Work out the finished part from the listing and answer in its coordinate system (mm). A direction names the side the tool comes from. Coordinates: 2 decimals unless noted, no trailing zeros. Loops run counter-clockwise (first coordinate to the right, second up) from the corner with the lowest first, then second, coordinate; pieces in that order, holes last. Notation, with made-up numbers: (71, 56) -> (85, 56) arc R12 ccw to (85, 68) -> close; hole circle Ø5 at (6, 18.25). An arc over 180 degrees is marked (long way). One line per question, with ' | ' between items.
```python
from build123d import *

# Parameters (mm, degrees)
F0_R          = 12.7
F1_DEPTH      = 25.4
F2_R          = 12.7
F3_R          = 12.69999
F4_R          = 17.8783824342
F5_DEPTH      = 1.27
F5_DEPTH_BACK = 2.032
F6_R          = 10.795
F7_DEPTH      = 38.1
F8_R          = 19.05
F9_DEPTH      = 15.24


# Not quite as in the source:
# - a fillet or chamfer that OpenCascade refuses, or shapes differently, is made with other operations: its cross-section is extruded or revolved along the edge and cut away or added
# - a fillet or chamfer is up to 0.001 mm smaller than in the source, because OpenCascade refuses the exact size


with BuildPart() as f1:
    # F0 (on Front) → F1 (new body)
    with BuildSketch(Plane.XZ):
        Circle(F0_R)
    extrude(amount=F1_DEPTH)

    # F2
    f2_edges = [f1.edges().sort_by_distance(p)[0] for p in [
        (-12.7, -25.4, 0),
    ]]
    fillet(f2_edges, radius=F2_R)

    # F3 (radius 12.7 in the source; OpenCascade refuses exactly that, so slightly less here)
    f3_edges = [f1.edges().sort_by_distance(p)[0] for p in [
        (-12.7, 0, 0),
    ]]
    fillet(f3_edges, radius=F3_R)

    # F4 (on Front) → F5 (join, two sides)
    with BuildSketch(Plane.XZ) as f5_sk:
        Circle(F4_R)
    extrude(amount=-F5_DEPTH)
    extrude(f5_sk.sketch, amount=F5_DEPTH_BACK)

    # F6 (on face) → F7 (join)
    with BuildSketch(Plane(origin=(0, 1.27, 0), x_dir=(-1, 0, 0), z_dir=(0, 1, 0))):
        Circle(F6_R)
    extrude(amount=F7_DEPTH)

    # F8 (on face) → F9 (join)
    with BuildSketch(Plane(origin=(0, 39.37, 0), x_dir=(-1, 0, 0), z_dir=(0, 1, 0))):
        Circle(F8_R)
    extrude(amount=F9_DEPTH)

    # F10: fillet of radius 12.7 on 1 edges, made by hand

    # F10_s1 → F10_t2 (revolve, cut)
    with BuildSketch(Plane.XY):
        with BuildLine():
            ThreePointArc((-19.05, 51.2667211869), (-16.7841147205, 44.0266072376), (-10.795, 39.37))
            Line((-10.795, 39.37), (-19.05, 39.37))
            Line((-19.05, 39.37), (-19.05, 51.2667211869))
        make_face()
    revolve(axis=Axis((0, 39.37, 0), (0, 1, 0)), mode=Mode.SUBTRACT)


solid = f1.part
```
1) The mould has two halves that part along Y. Classify faces 3 (the face through (8, -2.032, 0)), 4 (the face through (0, 54.61, 0)), 5 (the face through (15.12, 52.91, -11.59)): released by +Y, released by -Y, zero draft, split by the parting line, or undercut.
Check values:
face 3: undercut | face 4: released by +Y | face 5: zero draft
2) For faces 1 (the face through (8, 1.27, -8)), 2 (the face through (-14.188, -0.404, -10.879)), determine the directions among +Z, -Z, +X, -X, +Y, -Y from which every point of the face is accessible in a straight line to the end or side of a thin tool.
Check values:
face 1: none | face 2: -Y
3) Find section A-A (y = 27.5). Write down the section's boundary in (x, z) (3 decimals).
Check values:
outline: circle Ø21.59 at (0, 0)
4) Flat-ended cylindrical pins translate along their axes: pin 1 (8 mm diameter, centred on y = 7, z = 7, fed in from -X); pin 2 (10 mm diameter, centred on x = 11.5, y = 32.5, fed in from -Z); pin 3 (8 mm diameter, centred on y = 38, z = -4.5, fed in from -X). Find the tip coordinate at first contact, or state that the pin passes through.
Check values:
pin 1: stops at x = -10.37 | pin 2: stops at z = -8.62 | pin 3: stops at x = -14.48
5) Find the intervals of material crossed by line 1 along Y through (x, z) = (-3, 12.5), in increasing order.
Check values:
line 1: y = -2.03 to 1.27, 40.36 to 54.61
